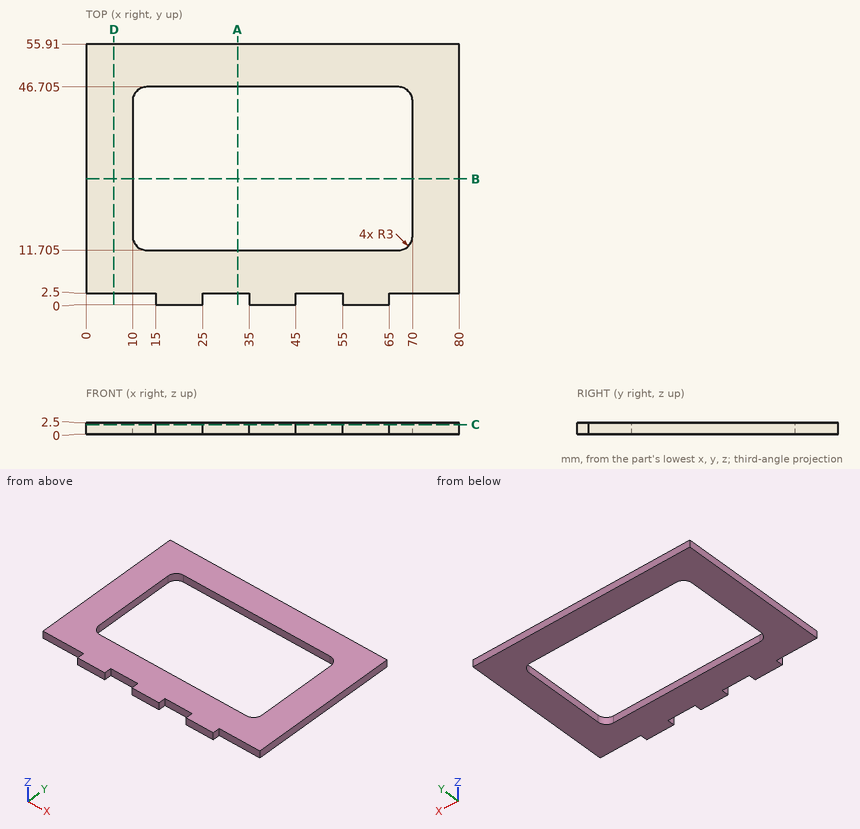
Can you work these out from the drawing? Everything is in mm from the part's minimum corner. Coordinates: 2 decimals unless noted, no trailing zeros. Loops run counter-clockwise (first coordinate to the right, second up) from the corner with the lowest first, then second, coordinate; pieces in that order, holes last. Notation, with made-up numbers: M 60.25,54.25 L 79.25,54.25 A23 ccw 79.25,70.25 Z; hole C -19,67.25 d10. An arc over 180 degrees is marked long. Put each result on its own line as item: value. Start each with the question number.
(1) Suppose I cut it at A-A on x = 32.5. Please give me the cut outline in (y, z) (3 decimals).
(2) Suppose I cut it at D-D on x = 6. Please give me the cut outline in (y, z).
(3) Suppose I cut it at B-B on y = 27. Please give me the cut outline in (x, z).
(4) Will these pins go through, and if not, where does the flat tip stop? P1, Ø1.5, axis at y = 16.5, z = 1.5, coming from the -X side; P2, Ø0.8, axis at x = 11, z = 1, coming from the -Y side; P3, Ø0.8, axis at y = 1, z = 1.5, coming from the -X side; P4, Ø0.8, axis at y = 1, z = 0.5, coming from the +X side.
(5) Suppose I cut it at C-C on z = 2.1. Please give me the cut outline in (x, y) (3 decimals).
(6) I need wall thicknesses on line 1 (X direction, y = 32.5, z = 1.5); line 2 (Y direction, x = 43.5, z = 2.3) (3 decimals); line 3 (Y direction, x = 7, z = 1.3). Which ranges of each line are inside material? Lowest first, please. Write a range as from..to.
Solutions:
1. outline: M 2.5,0 L 11.705,0 L 11.705,2.5 L 2.5,2.5 Z; M 46.705,0 L 55.91,0 L 55.91,2.5 L 46.705,2.5 Z
2. outline: M 2.5,0 L 55.91,0 L 55.91,2.5 L 2.5,2.5 Z
3. outline: M 0,0 L 10,0 L 10,2.5 L 0,2.5 Z; M 70,0 L 80,0 L 80,2.5 L 70,2.5 Z
4. P1: stops at x = 0
4. P2: stops at y = 2.5
4. P3: stops at x = 15
4. P4: stops at x = 65
5. outline: M 0,2.5 L 15,2.5 L 15,0 L 25,0 L 25,2.5 L 35,2.5 L 35,0 L 45,0 L 45,2.5 L 55,2.5 L 55,0 L 65,0 L 65,2.5 L 80,2.5 L 80,55.91 L 0,55.91 Z; hole M 10,14.705 A3 ccw 13,11.705 L 67,11.705 A3 ccw 70,14.705 L 70,43.705 A3 ccw 67,46.705 L 13,46.705 A3 ccw 10,43.705 Z
6. line 1: x = 0..10, 70..80
6. line 2: y = 0..11.705, 46.705..55.91
6. line 3: y = 2.5..55.91
